```python
from build123d import *


with BuildPart() as part:
    # Sketch1 → Diafisis (revolve)
    with BuildSketch(Plane.XY, mode=Mode.PRIVATE) as diafisis_sk:
        Polygon((0, 0), (6.8, 0), (7.5, -120), (0, -120), align=None)
    revolve(diafisis_sk.sketch.rotate(Axis((0, -124, 0), (0, 1, 0)), 90), axis=Axis((0, -124, 0), (0, 1, 0)))

    # Sketch2 → Union_proximal (revolve)
    with BuildSketch(Plane.XY):
        with BuildLine():
            Line((0, -6.8), (0, 6.8))
            ThreePointArc((0, 6.8), (6.8, 0), (0, -6.8))
        make_face()
    revolve(axis=Axis((0, -10.8, 0), (0, 1, 0)))

    # Sketch3 → Union_distal (revolve)
    with BuildSketch(Plane.XY):
        with BuildLine():
            Line((0, -127.5), (0, -112.5))
            ThreePointArc((0, -112.5), (7.5, -120), (0, -127.5))
        make_face()
    revolve(axis=Axis((0, -131.5, 0), (0, 1, 0)))


solid = part.part
```
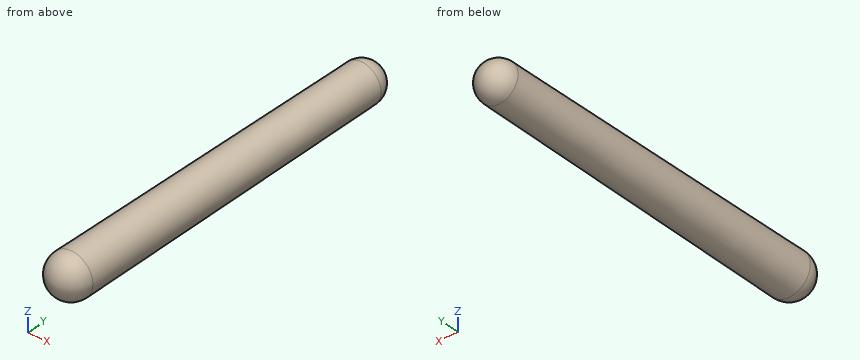
Verification items for the finished model (mm, model axes). Round coordinates to 2 decimals unless told otherwise and drop trailing zeros. Write each loop counter-clockwise with the first axis right and the second up, starting at its lowest first coordinate (ties: lowest second). Pieces come first, ordered by that corner, then holes.
1. Section check A-A on y = -20. Enter the section's corners in (x, z), plus the area to 3 significant figures.
2. Scan lines: L1, parallel to X at y = 0.5, z = 0.25; L2, parallel to Y at x = -6, z = -1; L3, parallel to Y at x = -0.5, z = 0. Record each from-to range of solid material in increasing order.
3. Gauge pin test, flat ends, axial feed: P1, Ø1.5, axis at x = 1, y = -64, coming from the +Z side; P2, Ø8, axis at x = -1, z = 3, coming from the -Y side; P3, Ø3, axis at y = -92, z = -1, coming from the +X side; P4, Ø2, axis at x = 4, z = 0, coming from the -Y side. Record the tip position at first contact, or that the pin passes through.
Answer:
1. outline: circle Ø13.83 at (0, 0)
1. area: 150 mm2
2. L1: x = -6.78 to 6.78
2. L2: y = -124.39 to 3.04
2. L3: y = -127.48 to 6.78
3. P1: stops at z = 7.17
3. P2: stops at y = -127.5
3. P3: stops at x = 7.34
3. P4: stops at y = -126.87
